Geometry check sheet. Reference: drawing and pictorial views, mm from the part's lowest x, y, z. Round coordinates to 2 decimals unless told otherwise and drop trailing zeros. Write each loop counter-clockwise with the first axis right and the second up, starting at its lowest first coordinate (ties: lowest second). Pieces come first, ordered by that corner, then holes. Notation, with made-up numbers: (82, -24) -> (99, -24) arc R32 cw to (99, 10) -> close; hole circle Ø5 at (19, 25.5). An arc over 180 degrees is marked (long way). Write item = value, one per line.
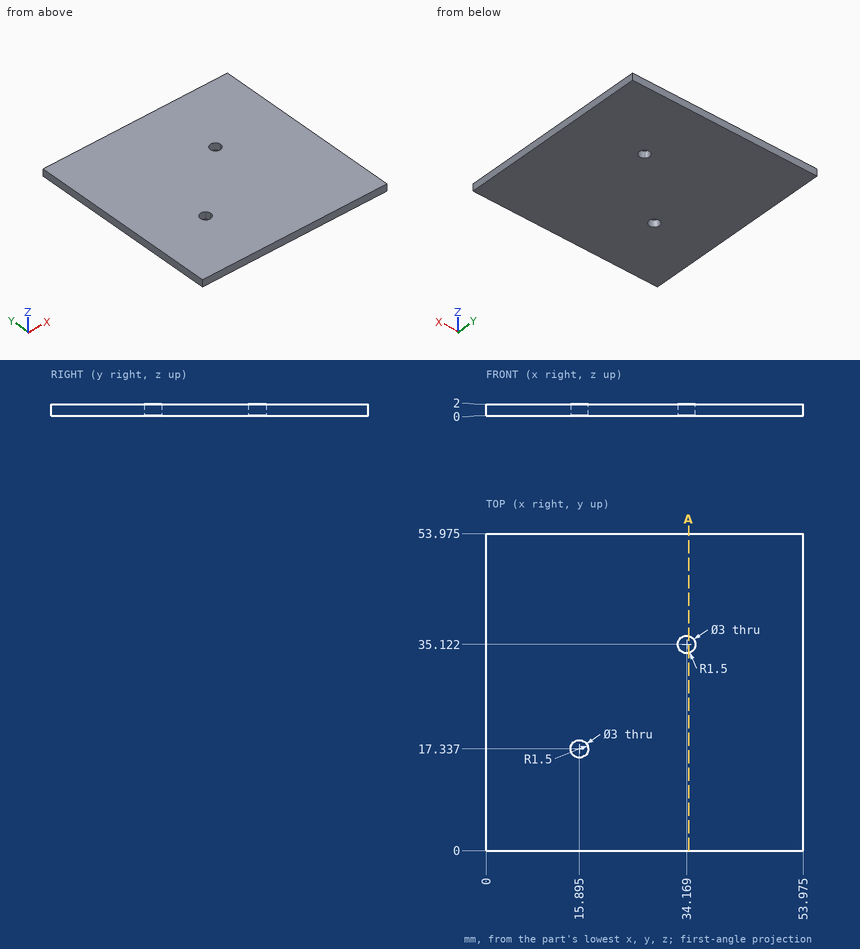
(1) Go/stop test with a flat-tipped pin: P1, Ø2.5, axis at x = 34.17, y = 35.12, coming from the +Z side. Record where the tip stops, or that it passes through.
Worked answers:
P1 = through
(2) Material ranges on L1, parallel to Y at x = 16.5, z = 0.3 (1 decimal); L2, parallel to X at y = 34, z = 1.4 (1 decimal); L3, parallel to Y at x = 17, z = 1.05 (1 decimal), recorded low to high. Write a range as [from, to].
Worked answers:
L1 = [0, 16], [18.7, 54]
L2 = [0, 33.2], [35.2, 54]
L3 = [0, 16.3], [18.4, 54]
(3) Sectioned sample at A-A on x = 34.5. Enter the section's corners in (y, z) (3 decimals).
Worked answers:
outline = (0, 0) -> (33.659, 0) -> (33.659, 2) -> (0, 2) -> close; (36.585, 0) -> (53.975, 0) -> (53.975, 2) -> (36.585, 2) -> close
